Input: part model. Units: mm. Frame: model coordinates. Coordinates: 2 decimals unless noted, no trailing zeros. Write each loop counter-clockwise with the first axis right and the second up, starting at its lowest first coordinate (ties: lowest second). Pieces come first, ordered by that corner, then holes. Notation, with made-up numbers: (-9.5, 16.5) -> (-1.5, 16.5) arc R34 ccw to (-1.5, 48.5) -> close; hole circle Ø9 at (-17.75, 35.25). An arc over 180 degrees is marked (long way). One line per question, with ' | ' between items. Start each with the question number.
```python
from build123d import *

# Parameters (mm, degrees)
F0_W     = 12.7
F0_H     = 12.7
F1_DEPTH = 12.7


with BuildPart() as f1:
    # F0 (on Front) → F1 (new body)
    with BuildSketch(Plane.XZ):
        with Locations((146.05, 146.05)):
            Rectangle(F0_W, F0_H)
        Polygon((139.7, 139.7), (139.7, 152.4), (120.65, 152.4), (120.65, 139.7), (107.95, 139.7), (107.95, 152.4), (95.25, 152.4), (95.25, 139.7), (82.55, 139.7), (82.55, 152.4), (69.85, 152.4), (69.85, 139.7), (57.15, 139.7), (57.15, 152.4), (44.45, 152.4), (44.45, 139.7), (31.75, 139.7), (31.75, 152.4), (19.05, 152.4), (19.05, 139.7), (6.35, 139.7), (6.35, 152.4), (-6.35, 152.4), (-6.35, 139.7), (-19.05, 139.7), (-19.05, 152.4), (-31.75, 152.4), (-31.75, 139.7), (-44.45, 139.7), (-44.45, 152.4), (-57.15, 152.4), (-57.15, 139.7), (-69.85, 139.7), (-69.85, 152.4), (-82.55, 152.4), (-82.55, 139.7), (-95.25, 139.7), (-95.25, 152.4), (-107.95, 152.4), (-107.95, 139.7), (-120.65, 139.7), (-120.65, 152.4), (-139.7, 152.4), (-139.7, 139.7), (-139.7, 127), (-152.4, 127), (-152.4, 114.3), (-139.7, 114.3), (-139.7, 101.6), (-152.4, 101.6), (-152.4, 88.9), (-139.7, 88.9), (-139.7, 76.2), (-152.4, 76.2), (-152.4, 63.5), (-139.7, 63.5), (-139.7, 50.8), (-152.4, 50.8), (-152.4, 38.1), (-139.7, 38.1), (-139.7, 25.4), (-152.4, 25.4), (-152.4, 12.7), (-139.7, 12.7), (-139.7, 0), (-152.4, 0), (-152.4, -12.7), (-139.7, -12.7), (-139.7, -25.4), (-152.4, -25.4), (-152.4, -38.1), (-139.7, -38.1), (-139.7, -50.8), (-152.4, -50.8), (-152.4, -63.5), (-139.7, -63.5), (-139.7, -76.2), (-152.4, -76.2), (-152.4, -88.9), (-139.7, -88.9), (-139.7, -101.6), (-152.4, -101.6), (-152.4, -114.3), (-139.7, -114.3), (-139.7, -127), (-152.4, -127), (-152.4, -139.7), (-139.7, -139.7), (-139.7, -152.4), (139.7, -152.4), (139.7, -139.7), (152.4, -139.7), (152.4, -127), (139.7, -127), (139.7, -114.3), (152.4, -114.3), (152.4, -101.6), (139.7, -101.6), (139.7, -88.9), (152.4, -88.9), (152.4, -76.2), (139.7, -76.2), (139.7, -63.5), (152.4, -63.5), (152.4, -50.8), (139.7, -50.8), (139.7, -38.1), (152.4, -38.1), (152.4, -25.4), (139.7, -25.4), (139.7, -12.7), (152.4, -12.7), (152.4, 0), (139.7, 0), (139.7, 12.7), (152.4, 12.7), (152.4, 25.4), (139.7, 25.4), (139.7, 38.1), (152.4, 38.1), (152.4, 50.8), (139.7, 50.8), (139.7, 63.5), (152.4, 63.5), (152.4, 76.2), (139.7, 76.2), (139.7, 88.9), (152.4, 88.9), (152.4, 101.6), (139.7, 101.6), (139.7, 114.3), (152.4, 114.3), (152.4, 127), (139.7, 127), align=None)
        with Locations((-146.05, 146.05)):
            Rectangle(F0_W, F0_H)
    extrude(amount=F1_DEPTH)


solid = f1.part
```
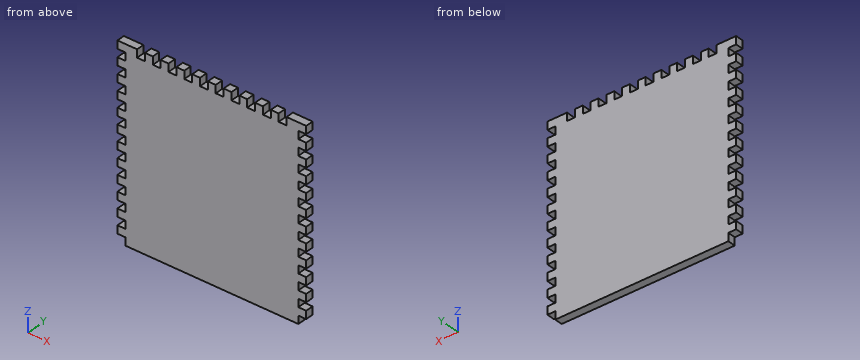
1) Ray query, line 1 (X direction, y = -1, z = 136.5); line 2 (Z direction, x = 58, y = -5). Return the intervals inside material, ascending.
2) Section B-B, the plane x = -114. Return loops of the section in (y, z).
3) First-contact query: P1, Ø4, axis at y = -4, z = 54, coming from the -X side; P2, Ø6.5, axis at x = -149, y = -7, coming from the -Z side. Flat tips, straight axial feed; report the tip coordinate or a pass-through.
4) Section A-A, the plane z = 82.5. Return loops of the section in (x, y), then the cut area to 3 significant figures.
Answer block:
1) line 1: x = -139.7 to 139.7 | line 2: z = -152.4 to 139.7
2) outline: (-12.7, -152.4) -> (0, -152.4) -> (0, 139.7) -> (-12.7, 139.7) -> close
3) P1: stops at x = -139.7 | P2: stops at z = -139.7
4) outline: (-139.7, -12.7) -> (139.7, -12.7) -> (139.7, 0) -> (-139.7, 0) -> close | area: 3,550 mm2
